Part model, mm, in its own coordinate system. Face numbers are marked on the shaded views. A direction names the side the tool comes from. Round coordinates to 2 decimals unless told otherwise and drop trailing zeros. Write each loop counter-clockwise with the first axis right and the second up, starting at its lowest first coordinate (ties: lowest second). Pieces come first, ordered by that corner, then holes. Notation, with made-up numbers: (13, 4.5) -> (47, 4.5) arc R5 cw to (47, 13.5) -> close; hole circle Ø5 at (35.5, -6.75). An arc over 180 degrees is marked (long way). Return JSON: item names as keys, results as strings. Group by question number.
(1) Saw through at A-A (z = 64). List the corners of the cut face in (x, y).
(2) Drill centre lines: L1, parallel to X at y = 79, z = 85.5; L2, parallel to X at y = -89, z = 63. Where is each one in solid material? Low to high. Write a range as from..to.
(3) Mould opens along Y. For the marked faces 3, 4 and 5 say: +Y half, -Y half, draft (parallel to the pull), parting line (faces both ways), or undercut.
(4) Drop a flat-ended pin along its axis: pin 1 Ø12.5 at (y, z) = (90, 65.5) entering from +X. Give the stop position or say it passes through.
(5) Saw through at B-B (y = 84.5). List the corners of the cut face in (x, z), plus the area to 3 significant figures.
(6) Tool access for the marked faces 1 and 2: list every direction of +Z, -Z, +X, -X, +Y, -Y with a clear straight run to the whole face (end or side of a thin tool).
(7) Saw through at C-C (x = -4). List the corners of the cut face in (y, z), plus the area to 3 significant figures.
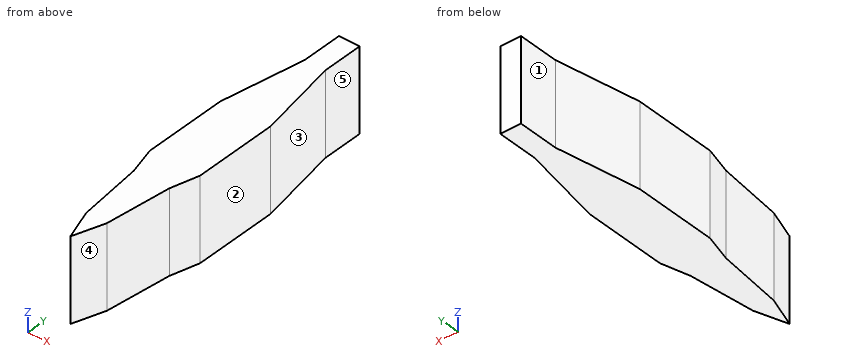
from build123d import *

# Parameters (mm, degrees)
F0_W     = 127
F0_H     = 203.2
F1_DEPTH = 101.6
F3_DEPTH = 50.8
F4_DEPTH = 127.001


with BuildPart() as f1:
    # F0 (on Top) → F1 (new body)
    with BuildSketch(Plane.XY):
        Rectangle(F0_W, F0_H)
    extrude(amount=F1_DEPTH)

    # F2 (on face) → F3 (cut)
    with BuildSketch(Plane.XY.offset(101.6)):
        Polygon((-6.35, -82.4402868748), (-10.8761594549, -42.4315269709), (-15.4023189098, -25.4), (-15.4023189098, 25.8809477091), (-6.35, 76.6328498721), (-6.35, 101.6), (-63.5, 101.6), (-63.5, -101.6), (0, -101.6), align=None)
        Polygon((15.4023189098, -25.4), (10.8761594549, -42.4315269709), (6.35, -82.4402868748), (0, -101.6), (63.5, -101.6), (63.5, 101.6), (6.35, 101.6), (6.35, 76.6328498721), (15.4023189098, 25.8809477091), align=None)
    extrude(amount=-F3_DEPTH, mode=Mode.SUBTRACT)

    # F4 (cut, through all): a face of the model
    f4_faces = [f1.faces().sort_by_distance(p)[0] for p in [
        (63.5, 0, 25.4),
    ]]
    extrude(f4_faces, amount=-F4_DEPTH, mode=Mode.SUBTRACT)


solid = f1.part
Computed values:
{
 "1": {"outline": "(-15.4, -25.4) -> (-10.88, -42.43) -> (-6.35, -82.44) -> (0, -101.6) -> (6.35, -82.44) -> (10.88, -42.43) -> (15.4, -25.4) -> (15.4, 25.88) -> (6.35, 76.63) -> (6.35, 101.6) -> (-6.35, 101.6) -> (-6.35, 76.63) -> (-15.4, 25.88) -> close"},
 "2": {"L1": "-6.35..6.35", "L2": "-4.18..4.18"},
 "3": {"face 3": "+Y half", "face 4": "-Y half", "face 5": "draft"},
 "4": {"pin 1": "x = 6.35"},
 "5": {"outline": "(-6.35, 50.8) -> (6.35, 50.8) -> (6.35, 101.6) -> (-6.35, 101.6) -> close", "area": "645 mm2"},
 "6": {"face 1": "+Z, -Z, -X, +Y", "face 2": "+Z, -Z, +X, +Y, -Y"},
 "7": {"outline": "(-89.53, 50.8) -> (101.6, 50.8) -> (101.6, 101.6) -> (-89.53, 101.6) -> close", "area": "9,710 mm2"}
}
